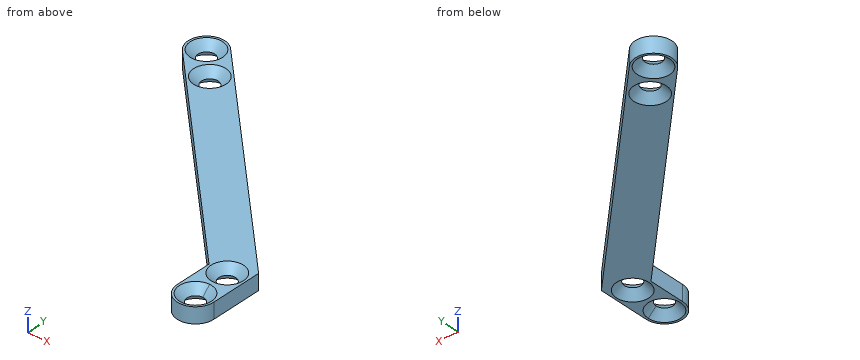
Autodesk Inventor part; units mm, degrees
ref_plane "YZ Plane" through (0, 0, 0) normal (1, 0, 0) x (0, 1, 0)
ref_plane "XZ Plane" through (0, 0, 0) normal (0, 1, 0) x (-1, 0, 0)
ref_plane "XY Plane" through (0, 0, 0) normal (0, 0, 1) x (1, 0, 0)
sketch "Эскиз1" plane through (0, 0, 0) normal (0, 0, 1) x (1, 0, 0)
  circle A0 centre (-6.3231, 9.8469) radius 1.6
  circle A1 centre (-6.3231, 16.8469) radius 1.6
  line L0 (-6.3231, 9.8469) -> (-6.3231, 16.8469)
  circle A2 centre (-6.3231, 16.8469) radius 3.5
  circle A3 centre (-6.3231, 9.8469) radius 3.5
  line L1 (-9.8231, 9.8469) -> (-9.8231, 16.8469)
  line L2 (-2.8231, 9.8469) -> (-2.8231, 16.8469)
  line L3 (-9.8231, 16.8469) -> (-41.6784, 48.7022)
  line L4 (-9.8231, 16.8469) -> (40.1769, 16.8469) construction
  line L5 (-36.7287, 53.652) -> (-41.6784, 48.7022)
  line L6 (-39.2035, 51.1771) -> (-41.6784, 53.652) construction
  circle A4 centre (-41.6784, 53.652) radius 3.5
  line L7 (-36.7287, 53.652) -> (-2.8231, 19.7464)
  line L8 (-2.8231, 19.7464) -> (-2.8231, 16.8469)
  circle A5 centre (-41.6784, 53.652) radius 1.6
  line L9 (-41.6784, 53.652) -> (-46.6281, 58.6017) construction
  circle A6 centre (-46.6281, 58.6017) radius 3.5
  circle A7 centre (-46.6281, 58.6017) radius 1.6
  line L10 (-41.6784, 48.7022) -> (-49.103, 56.1268)
  line L11 (-36.7287, 53.652) -> (-44.1533, 61.0766)
  point P0 (0, 0)
  dimension "d0" = 3.2
  dimension "d1" = 3.2
  dimension "d2" = 7
  dimension "d3" = 7
  dimension "d4" = 7
  dimension "d8" = 135
  dimension "d9" = 45.0502
  dimension "d10" = 3.5
  dimension "d11" = 7
  dimension "d12" = 3.2
  dimension "d13" = 7
  dimension "d14" = 3.2
extrude "Выдавливание1" add sketch "Эскиз1" along normal blind 3
chamfer "Фаска1" distance 1.5 angle 45 4 edges at (-7.9231, 9.8469, 3) (-7.9231, 16.8469, 3) (-43.2784, 53.652, 3) (-48.2281, 58.6017, 3)
chamfer "Фаска2" distance 1.5 angle 45 4 edges at (-7.9231, 9.8469, 0) (-7.9231, 16.8469, 0) (-43.2784, 53.652, 0) (-48.2281, 58.6017, 0)
properties part number "каркас1"
Can you work these out from the model? Positions are in its coordinate system, mm. Coordinates: 2 decimals unless noted, no trailing zeros. Loops run counter-clockwise (first coordinate to the right, second up) from the corner with the lowest first, then second, coordinate; pieces in that order, holes last. Notation, with made-up numbers: (-0.5, 17.25) -> (22.5, 17.25) arc R19 cw to (22.5, 37.25) -> close; hole circle Ø5 at (14, 13). An arc over 180 degrees is marked (long way). Put each result on its own line as item: value. Start each with the question number.
Q1. I want a section at B-B (x = -10.5). Write out the boundary of the cut face in (y, z).
Q2. I'm going to push flat-ended pins straight in: P1, Ø3, axis at x = -6.32, y = 16.85, coming from the +Z side; P2, Ø1.5, axis at x = -31.5, z = 1.5, coming from the -Y side; P3, Ø1, axis at x = -26, z = 2, coming from the +Y side; P4, Ø1.5, axis at y = 13, z = 2, coming from the -X side. Where does each tip first touch, or does it pass through?
Q3. If I drill on line 1 (X direction, y = 59, z = 1.55); line 2 (X direction, y = 58, z = 1.3); line 3 (Y direction, x = -47, z = 2.3), over which ranges is the centre line in solid material (lowest first)? Write a range as [from, to].
Q4. I want a section at A-A (z = 0.95). Count the separate pieces of the cut face and the enclosed holes in it, plus the area to 3 significant figures.
Q5. I want a section at C-C (y = 38). Write out the boundary of the cut face in (x, z).
Taken from the geometry:
1. outline: (17.52, 0) -> (27.42, 0) -> (27.42, 3) -> (17.52, 3) -> close
2. P1: passes through
2. P2: stops at y = 37.77
2. P3: stops at y = 43.42
2. P4: stops at x = -9.82
3. line 1: x = [-50.11, -48.23], [-45.03, -42.08]
3. line 2: x = [-50.08, -48.32], [-44.93, -41.08]
3. line 3: y = [54.02, 56.23], [60.97, 62.08]
4. separate pieces: 1
4. enclosed holes: 4
4. area: 439 mm2
5. outline: (-30.98, 0) -> (-21.08, 0) -> (-21.08, 3) -> (-30.98, 3) -> close
